Could you check a few things on this model? Use its own coordinates, in mm. A direction names the side the tool comes from. Round coordinates to 2 decimals unless told otherwise and drop trailing zeros. Order: outer loops, then holes, each group sorted by start corner. A loop starts at its lowest first (then second) coordinate and runs counter-clockwise, first axis right, second up. Notation, with made-up numbers: (46.25, -35) - (66.25, -35) arc R23 ccw to (66.25, -12) - close; hole circle Ø3 at (0, -7). An arc over 180 degrees is marked (long way). Use one line per item in the form item = value.
from build123d import *

# Parameters (mm, degrees)
F0_R      = 26.5
F1_DEPTH  = 45
F2_R      = 20.5
F3_DEPTH  = 30
F4_R      = 2.5
F5_DEPTH  = 45.001
F7_DEPTH  = 10
F9_DEPTH  = 45.001
F10_R     = 15
F11_DEPTH = 6
F12_R     = 4.6840080941
F13_DEPTH = 10


with BuildPart() as f1:
    # F0 (on Front) → F1 (new body)
    with BuildSketch(Plane.XZ):
        Circle(F0_R)
    extrude(amount=F1_DEPTH)

    # F2 (on face) → F3 (cut)
    with BuildSketch(Plane.XZ.offset(45)):
        Circle(F2_R)
    extrude(amount=-F3_DEPTH, mode=Mode.SUBTRACT)

    # F4 (on face) → F5 (cut, through all)
    with BuildSketch(Plane(origin=(0, 0, 0), x_dir=(-1, 0, 0), z_dir=(0, 1, 0))):
        Circle(F4_R)
    extrude(amount=-F5_DEPTH, mode=Mode.SUBTRACT)

    # F6 (on face) → F7 (cut)
    with BuildSketch(Plane.XZ.offset(15)):
        with BuildLine():
            Line((3.4260696722, 2.917541191), (-3.4260696722, 2.917541191))
            ThreePointArc((-3.4260696722, 2.917541191), (0, -4.5), (3.4260696722, 2.917541191))
        make_face()
    extrude(amount=-F7_DEPTH, mode=Mode.SUBTRACT)

    # F8 (on face) → F9 (cut, through all)
    with BuildSketch(Plane(origin=(0, 0, 0), x_dir=(-1, 0, 0), z_dir=(0, 1, 0))):
        with BuildLine():
            Line((-25.9593629808, 5.325549139), (-12.0217161029, 23.6162728207))
            ThreePointArc((-12.0217161029, 23.6162728207), (-21.077908703, 16.061499454), (-25.9593629808, 5.325549139))
        make_face()
        with BuildLine():
            ThreePointArc((10.9685281987, 24.1234613842), (-0.584475192, 26.4935537207), (-12.0217161029, 23.6162728207))
            Line((-12.0217161029, 23.6162728207), (10.9685281987, 24.1234613842))
        make_face()
        with BuildLine():
            ThreePointArc((25.6992470496, 6.4651914964), (20.3490800596, 16.9754216657), (10.9685281987, 24.1234613842))
            Line((10.9685281987, 24.1234613842), (25.6992470496, 6.4651914964))
        make_face()
        with BuildLine():
            ThreePointArc((26.5, 0), (26.2990498575, 3.257295902), (25.6992470496, 6.4651914964))
            Line((25.6992470496, 6.4651914964), (21.077908703, -16.061499454))
            ThreePointArc((21.077908703, -16.061499454), (25.1079129024, -8.4760078861), (26.5, 0))
        make_face()
        with BuildLine():
            ThreePointArc((0.584475192, -26.4935537207), (12.0217161029, -23.6162728207), (21.077908703, -16.061499454))
            Line((21.077908703, -16.061499454), (0.584475192, -26.4935537207))
        make_face()
        with BuildLine():
            Line((0.584475192, -26.4935537207), (-20.3490800596, -16.9754216657))
            ThreePointArc((-20.3490800596, -16.9754216657), (-10.9685281987, -24.1234613842), (0.584475192, -26.4935537207))
        make_face()
        with BuildLine():
            Line((-20.3490800596, -16.9754216657), (-25.9593629808, 5.325549139))
            ThreePointArc((-25.9593629808, 5.325549139), (-25.6992470496, -6.4651914964), (-20.3490800596, -16.9754216657))
        make_face()
    extrude(amount=-F9_DEPTH, mode=Mode.SUBTRACT)

    # F10 (on face) → F11 (join)
    with BuildSketch(Plane(origin=(0, 0, 0), x_dir=(-1, 0, 0), z_dir=(0, 1, 0))):
        Polygon((-12.0217161029, 23.6162728207), (-25.9593629808, 5.325549139), (-20.3490800596, -16.9754216657), (0.584475192, -26.4935537207), (21.077908703, -16.061499454), (25.6992470496, 6.4651914964), (10.9685281987, 24.1234613842), align=None)
        Circle(F10_R, mode=Mode.SUBTRACT)
    extrude(amount=F11_DEPTH)

    # F12 (on face) → F13 (cut)
    with BuildSketch(Plane.XZ.offset(15)):
        with Locations((11.9633907452, 0)):
            Circle(F12_R)
        with Locations((3.6968910506, 11.3778607252)):
            Circle(F12_R)
        with Locations((-9.6785864232, 7.0319046475)):
            Circle(F12_R)
        with Locations((-9.6785864232, -7.0319046475)):
            Circle(F12_R)
        with Locations((3.6968910506, -11.3778607252)):
            Circle(F12_R)
    extrude(amount=-F13_DEPTH, mode=Mode.SUBTRACT)


solid = f1.part
Item 1: Imagine slicing it at D-D on x = -6. Please give me the cut outline in (y, z), plus the area to 3 significant figures.
Found:
outline = (-45, -23.74) - (6, -23.74) - (6, -13.75) - (0, -13.75) - (0, 13.75) - (6, 13.75) - (6, 24.01) - (-45, 24.01) - (-45, 19.6) - (-15, 19.6) - (-15, 9.93) - (-5, 9.93) - (-5, 4.13) - (-15, 4.13) - (-15, -4.13) - (-5, -4.13) - (-5, -9.93) - (-15, -9.93) - (-15, -19.6) - (-45, -19.6) - close
area = 978 mm2
Item 2: Imagine slicing it at A-A on y = 2.5. Please give me the cut outline in (x, z).
Found:
outline = (-25.7, 6.47) - (-21.08, -16.06) - (-0.58, -26.49) - (20.35, -16.98) - (25.96, 5.33) - (12.02, 23.62) - (-10.97, 24.12) - close; hole circle Ø30 at (0, 0)
Item 3: If we mould it in two halves opening along X, with no side actions, what happens to faces 4 (the face through (10.029, -19.857, -21.668)), 5 (the face through (0, -10, 2.918)), 6 (the face through (0, 6, 16)), 7 (the face through (0.54, -2.46, -2.44))? For each: released by +X, released by -X, zero draft, split by the parting line, or undercut.
Found:
face_4 = released by +X
face_5 = undercut
face_6 = zero draft
face_7 = undercut
Item 4: I need wall thicknesses on L1, parallel to X at y = -8, z = 10.5; L2, parallel to X at y = -33, z = 17; L3, parallel to Z at x = 0, y = 2.95. Which ranges of each line are inside material? Lowest first, please.
Found:
L1 = -22.33 to -12.83, -6.53 to -0.9, 8.3 to 22.02
L2 = -16.91 to -11.46, 11.46 to 17.06
L3 = -26.23 to -15, 15 to 23.88
Item 5: Will these pins go through, and if not, where does the flat tip stop? P1, Ø2, axis at y = -2, z = 6.5, coming from the -X side; P2, Ø4, axis at x = 8, y = -19, coming from the -Z side; P3, Ø15, axis at x = 2, z = 5, coming from the +Y side.
Found:
P1 = -25.7
P2 = -23.5
P3 = 0
Item 6: For faces 1 (the face through (14.985, 2.958, 0.66)), 2 (the face through (-10.69, -19.86, -21.35)), 3 (the face through (-2, -5, -2)), which set-ups out of +Z, -Z, +X, -X, +Y, -Y let a thin tool reach every point of the face, with its end or its side?
Found:
face_1 = +Y
face_2 = -Z, -X, +Y, -Y
face_3 = -Y
Item 7: Imagine slicing it at B-B on z = 0. Please give me the cut outline in (x, y).
Found:
outline = (-24.37, -45) - (-20.5, -45) - (-20.5, -15) - (-4.5, -15) - (-4.5, -5) - (-2.5, -5) - (-2.5, 0) - (-15, 0) - (-15, 6) - (-24.37, 6) - close; (2.5, -5) - (4.5, -5) - (4.5, -15) - (7.28, -15) - (7.28, -5) - (16.65, -5) - (16.65, -15) - (20.5, -15) - (20.5, -45) - (24.62, -45) - (24.62, 6) - (15, 6) - (15, 0) - (2.5, 0) - close
Item 8: Imagine slicing it at C-C on y = -6. Please give me the cut outline in (x, z).
Found:
outline = (-25.7, 6.47) - (-21.08, -16.06) - (-0.58, -26.49) - (20.35, -16.98) - (25.96, 5.33) - (12.02, 23.62) - (-10.97, 24.12) - close; hole circle Ø9.37 at (-9.68, -7.03); hole circle Ø9.37 at (-9.68, 7.03); hole (-3.43, 2.92) arc R4.5 ccw (long way) to (3.43, 2.92) - close; hole circle Ø9.37 at (3.7, -11.38); hole circle Ø9.37 at (3.7, 11.38); hole circle Ø9.37 at (11.96, 0)
